Design review of the part built by this model. Coordinates are the model's own, in mm. Round coordinates to 2 decimals unless told otherwise and drop trailing zeros. Write each loop counter-clockwise with the first axis right and the second up, starting at its lowest first coordinate (ties: lowest second). Pieces come first, ordered by that corner, then holes. Notation, with made-up numbers: M 30,85 L 79,85 A25 ccw 79,121 Z; hole C -2,88 d11. An arc over 180 degrees is marked long. Use CSV: the item, a comma, the result in double quotes.
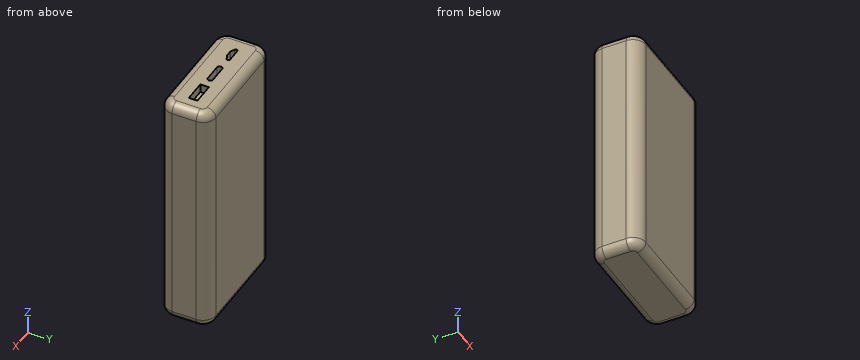
from build123d import *

# Parameters (mm, degrees)
ESQUISSE1_W             = 68
ESQUISSE1_H             = 29
BOSS_EXTRU_1_DEPTH      = 140
CONG_1_R                = 7.5
CONG_2_R                = 5
ESQUISSE2_W             = 12.5
ESQUISSE2_H             = 5
ENL_V_MAT_EXTRU_1_DEPTH = 5
CONG_3_R                = 1


with BuildPart() as part:
    # Esquisse1 → Boss.-Extru.1 (new body)
    with BuildSketch(Plane.XY):
        Rectangle(ESQUISSE1_W, ESQUISSE1_H)
    extrude(amount=BOSS_EXTRU_1_DEPTH)

    # Congé1
    cong_1_edges = [part.edges().sort_by_distance(p)[0] for p in [
        (-34, 14.5, 70),
        (34, 14.5, 70),
        (34, -14.5, 70),
        (-34, -14.5, 70),
    ]]
    fillet(cong_1_edges, radius=CONG_1_R)

    # Congé2
    cong_2_edges = [part.edges().sort_by_distance(p)[0] for p in [
        (34, 0, 0),
        (34, 0, 140),
        (-34, 0, 0),
        (0, 14.5, 0),
        (0, -14.5, 0),
        (-31.803300859, 12.303300859, 0),
        (-31.803300859, -12.303300859, 0),
        (31.803300859, 12.303300859, 0),
        (31.803300859, -12.303300859, 0),
        (0, -14.5, 140),
        (-34, 0, 140),
        (0, 14.5, 140),
        (-31.803300859, 12.303300859, 140),
        (-31.803300859, -12.303300859, 140),
        (31.803300859, 12.303300859, 140),
        (31.803300859, -12.303300859, 140),
    ]]
    fillet(cong_2_edges, radius=CONG_2_R)

    # Esquisse2 → Enlèv. mat.-Extru.1 (cut)
    with BuildSketch(Plane.XY.offset(140)):
        Polygon((-12.75, 1.5), (-22.75, 1.5), (-22.75, 0), (-19.52732972, -1.5), (-15.97267028, -1.5), (-12.75, 0), align=None)
        with BuildLine():
            Line((5, 1.5), (-5, 1.5))
            ThreePointArc((-5, 1.5), (-6.5, 0), (-5, -1.5))
            Line((-5, -1.5), (5, -1.5))
            ThreePointArc((5, -1.5), (6.5, 0), (5, 1.5))
        make_face()
        with Locations((17.75, 0)):
            Rectangle(ESQUISSE2_W, ESQUISSE2_H)
    extrude(amount=-ENL_V_MAT_EXTRU_1_DEPTH, mode=Mode.SUBTRACT)

    # Congé3
    # the kernel refuses this fillet: 1 mm, written as the material it adds along each edge
    with BuildSketch(Plane(origin=(-15.97267028, -1.5, 140), x_dir=(0.9066045100812768, 0.4219813530243817, 0), z_dir=(0, 0, -1)), Plane(origin=(-19.52732972, -1.5, 140), x_dir=(1, 0, 0), z_dir=(0, 0, -1))) as cong_3_piece_1:
        with BuildLine():
            CenterArc((CONG_3_R * 0.221326106591, -CONG_3_R), CONG_3_R, 90, 24.959741925)
            Line((-CONG_3_R * 0.200655246434, -CONG_3_R * 0.0933954899187), (0, 0))
            Line((0, 0), (CONG_3_R * 0.221326106591, 0))
        make_face()
    extrude(amount=5.553315266)
    with BuildSketch(Plane(origin=(-22.75, 0, 140), x_dir=(0.9066045100812758, -0.42198135302438383, 0), z_dir=(0, 0, -1))) as cong_3_piece_2:
        with BuildLine():
            CenterArc((CONG_3_R * 0.637564274773, -CONG_3_R), CONG_3_R, 90, 65.040258075)
            Line((-CONG_3_R * 0.269040235309, -CONG_3_R * 0.578018646976), (0, 0))
            Line((0, 0), (CONG_3_R * 0.637564274773, 0))
        make_face()
    extrude(amount=6.593910687)
    with BuildSketch(Plane(origin=(-22.75, 1.5, 140), x_dir=(0, -1, 0), z_dir=(0, 0, -1)), Plane(origin=(-12.75, 1.5, 140), x_dir=(-1, 0, 0), z_dir=(0, 0, -1))) as cong_3_piece_3:
        with BuildLine():
            CenterArc((CONG_3_R, -CONG_3_R), CONG_3_R, 90, 90)
            Line((0, -CONG_3_R), (0, 0))
            Line((0, 0), (CONG_3_R, 0))
        make_face()
    extrude(amount=7.5)
    with BuildSketch(Plane(origin=(-12.75, 0, 140), x_dir=(-0.906604510081276, -0.4219813530243839, 0), z_dir=(0, 0, -1))) as cong_3_piece_4:
        with BuildLine():
            CenterArc((CONG_3_R * 0.637564274773, CONG_3_R), CONG_3_R, 204.959741925, 65.040258075)
            Line((-CONG_3_R * 0.269040235309, CONG_3_R * 0.578018646976), (0, 0))
            Line((0, 0), (CONG_3_R * 0.637564274773, 0))
        make_face()
    extrude(amount=6.593910687)


solid = part.part
1) For pin 1 Ø1.5 at (x, y) = (2, -0.5) entering from +Z; pin 2 Ø1.5 at (x, z) = (-18, 137) entering from -Y; pin 3 Ø5.5 at (x, z) = (17, 138.5) entering from +Y, all flat-tipped, find the tip position at first contact; note any pin that passes through.
Answers:
pin 1,"z = 135"
pin 2,"y = -14.34"
pin 3,"y = 14.44"
2) Wall thickness on line 1 along Y through (x, z) = (27, 129.5); line 2 along Z through (x, y) = (21, 1.5); line 3 along X through (y, z) = (11.75, 134): over which ranges is each line inside the solid? List them lowest first. Write a range as [from, to].
Answers:
line 1,"[-14.48, 14.48]"
line 2,"[0, 135]"
line 3,"[-32.3, 32.3]"
3) Add section A-A on z = 30. Write out the cut boundary in (x, y), then the cut area to 3 significant figures.
Answers:
outline,"M -34,-7 A7.5 ccw -26.5,-14.5 L 26.5,-14.5 A7.5 ccw 34,-7 L 34,7 A7.5 ccw 26.5,14.5 L -26.5,14.5 A7.5 ccw -34,7 Z"
area,"1,920 mm²"
